Geometry: final body of the model. Coordinates: model frame, mm. Coordinates: 2 decimals unless noted, no trailing zeros. Loops run counter-clockwise (first coordinate to the right, second up) from the corner with the lowest first, then second, coordinate; pieces in that order, holes last. Notation, with made-up numbers: (85.5, -10) - (143.5, -10) arc R34 ccw to (143.5, 23) - close; hole circle Ø2 at (79, 69). An arc over 180 degrees is marked (long way). Put each result on its own line as item: value. Start each with the question number.
1) Section D-D on z = 9.5. Output: boundary loops of the cut face in (x, y) (3 decimals), and give its area (3 significant figures).
2) Draft query along Y for faces 1 (the cylindrical face through (-0.327, 2.494, 5.443)), 2 (the conical face through (2.27, 10.2, 0.16)), 3 (the flat face through (2, 2, 0)). Return one class per face: +Y half, -Y half, draft (parallel to the pull), parting line (faces both ways), or undercut.
3) Material intervals for line 1 along Y through (x, z) = (0, 7) (3 decimals); line 2 along X through (y, z) = (-3, 10); line 3 along X through (y, z) = (10.5, 6.5), sorted ascending. Write a range as from..to.
4) Contact query for flat-ended pins moving along their axis: pin 1 Ø1 at (y, z) = (6, 3) entering from -X; pin 2 Ø1 at (x, z) = (-9.5, 4.5) entering from -Y; pin 3 Ø4 at (y, z) = (9.5, 6.5) entering from -X. Output: stop coordinate, or through.
5) Section C-C on z = 4.5. Output: boundary loops of the cut face in (x, y) (3 decimals).
6) Section A-A on y = 0. Output: boundary loops of the cut face in (x, z) (3 decimals), and give its area (3 significant figures).
```python
from build123d import *

# Parameters (mm, degrees)
SKETCH1_R           = 11.975
BOSS_EXTRUDE1_DEPTH = 11.04
SKETCH2_R           = 2.515
CUT_EXTRUDE1_DEPTH  = 11.04


with BuildPart() as part:
    # Sketch1 → Boss-Extrude1 (new body)
    with BuildSketch(Plane.XY):
        Circle(SKETCH1_R)
    extrude(amount=BOSS_EXTRUDE1_DEPTH)

    # Sketch2 → Cut-Extrude1 (cut)
    with BuildSketch(Plane.XY):
        Circle(SKETCH2_R)
    extrude(amount=CUT_EXTRUDE1_DEPTH, mode=Mode.SUBTRACT)

    # Sketch3 → Cut-Revolve4 (revolve, cut)
    with BuildSketch(Plane(origin=(0, 0, 0), x_dir=(1, 0, 0), z_dir=(0, 1, 0))):
        Polygon((-7.292190974, 0), (-10.347240804, 0), (-11.975, -2.52), (-11.975, -8.52), (-10.347240804, -11.04), (-6.458257889, -11.04), (-5.810000317, -18.325003181), (-21.89407965, -6.340173639), (-13.168343432, 5.370083322), align=None)
    revolve(axis=Axis((0, 0, -5.854641455), (0, 0, 1)), mode=Mode.SUBTRACT)


solid = part.part
```
Answer block:
1. outline: circle Ø22.684 at (0, 0); hole circle Ø5.03 at (0, 0)
1. area: 384 mm²
2. face 1: undercut
2. face 2: parting line
2. face 3: draft
3. line 1: y = -11.975..-2.515, 2.515..11.975
3. line 2: x = -10.6..10.6
3. line 3: x = -5.76..5.76
4. pin 1: stops at x = -10.64
4. pin 2: stops at y = -7.9
4. pin 3: stops at x = -9.34
5. outline: circle Ø23.95 at (0, 0); hole circle Ø5.03 at (0, 0)
6. outline: (-11.975, 2.52) - (-10.347, 0) - (-2.515, 0) - (-2.515, 11.04) - (-10.347, 11.04) - (-11.975, 8.52) - close; (2.515, 0) - (10.347, 0) - (11.975, 2.52) - (11.975, 8.52) - (10.347, 11.04) - (2.515, 11.04) - close
6. area: 201 mm²
